```python
from build123d import *

# Parameters (mm, degrees)
SKETCH1_W           = 25
SKETCH1_H           = 40
BOSS_EXTRUDE1_DEPTH = 3
SKETCH2_W           = 3
SKETCH2_H           = 10
BOSS_EXTRUDE2_DEPTH = 3
SKETCH3_R           = 7.5
CUT_EXTRUDE1_DEPTH  = 4


with BuildPart() as part:
    # Sketch1 → Boss-Extrude1 (new body)
    with BuildSketch(Plane(origin=(0, 0, 0), x_dir=(1, 0, 0), z_dir=(0, 1, 0))):
        Rectangle(SKETCH1_W, SKETCH1_H)
    extrude(amount=BOSS_EXTRUDE1_DEPTH)

    # Sketch2 → Boss-Extrude2 (add)
    with BuildSketch(Plane(origin=(0, 3, 0), x_dir=(1, 0, 0), z_dir=(0, 1, 0))):
        with Locations((14, -15)):
            Rectangle(SKETCH2_W, SKETCH2_H)
        with Locations((14, 5)):
            Rectangle(SKETCH2_W, SKETCH2_H)
        with Locations((-14, -15)):
            Rectangle(SKETCH2_W, SKETCH2_H)
        with Locations((-14, 5)):
            Rectangle(SKETCH2_W, SKETCH2_H)
    extrude(amount=-BOSS_EXTRUDE2_DEPTH)

    # Sketch3 → Cut-Extrude1 (cut, through all)
    with BuildSketch(Plane(origin=(0, 3, 0), x_dir=(1, 0, 0), z_dir=(0, 1, 0))):
        with Locations((0, -7)):
            Circle(SKETCH3_R)
    extrude(amount=-CUT_EXTRUDE1_DEPTH, mode=Mode.SUBTRACT)


solid = part.part
```
For this review, take the finished solid that the model builds, in its own axes (mm). A direction names the side the tool comes from. Round coordinates to 2 decimals unless told otherwise and drop trailing zeros. Write each loop counter-clockwise with the first axis right and the second up, starting at its lowest first coordinate (ties: lowest second). Pieces come first, ordered by that corner, then holes. Notation, with made-up numbers: (71.5, 10) -> (92.5, 10) arc R17 ccw to (92.5, 43) -> close; hole circle Ø2 at (53, -29). An arc over 180 degrees is marked (long way). Use one line per item in the form item = value.
1) To check wall thickness, follow L1, parallel to Z at x = 0, y = 0.65; L2, parallel to X at y = 1.75, z = 7; L3, parallel to Z at x = -4, y = 2.1. State the ranges of each line that lie inside material, in increasing order. Write a range as from..to.
Found:
L1 = -20..-0.5, 14.5..20
L2 = -12.5..-7.5, 7.5..12.5
L3 = -20..0.66, 13.34..20
2) Take a section at C-C, the plane z = 7. Write out the cut boundary in (x, y), and give its area (3 significant figures).
Found:
outline = (-12.5, 0) -> (-7.5, 0) -> (-7.5, 3) -> (-12.5, 3) -> close; (7.5, 0) -> (12.5, 0) -> (12.5, 3) -> (7.5, 3) -> close
area = 30.0 mm2
3) Mouldability with a two-part tool opening along Z and no side actions: class faces 5 (the flat face through (-14, 2, 10)), 6 (the flat face through (0, 2, 20)), 7 (the flat face through (0, 3, -5)), 8 (the flat face through (14, 2, -10)) as +Z half, -Z half, draft (parallel to the pull), parting line (faces both ways), or undercut.
Found:
face_5 = undercut
face_6 = +Z half
face_7 = draft
face_8 = -Z half
4) Take a section at A-A, the plane x = 0. Write out the cut boundary in (y, z).
Found:
outline = (0, -20) -> (3, -20) -> (3, -0.5) -> (0, -0.5) -> close; (0, 14.5) -> (3, 14.5) -> (3, 20) -> (0, 20) -> close
5) Clearance check with flat-ended pins moving along their axes: pin 1 (0.9 mm diameter, centred on y = 1, z = 3.5, fed in from -X); pin 2 (1.5 mm diameter, centred on y = 1.5, z = -13, fed in from +X); pin 3 (0.9 mm diameter, centred on x = 14, y = 2, fed in from -Z). State where each tip first meets the part, or that it passes through.
Found:
pin_1 = -12.5
pin_2 = 12.5
pin_3 = -10
6) Tool access review of faces 1 (the flat face through (-14, 2, -10)), 2 (the flat face through (12.5, 1, 5)), 3 (the flat face through (-12.5, 1, 5)), 4 (the flat face through (12.5, 1, -15)): name each direction out of +Z, -Z, +X, -X, +Y, -Y from which nothing blocks a thin tool from reaching the whole face with its end or side.
Found:
face_1 = -Z, -X, +Y, -Y
face_2 = +X, +Y, -Y
face_3 = -X, +Y, -Y
face_4 = -Z, +X, +Y, -Y
7) Take a section at B-B, the plane y = 0.95. Write out the cut boundary in (x, z), and give its area (3 significant figures).
Found:
outline = (-15.5, -10) -> (-12.5, -10) -> (-12.5, -20) -> (12.5, -20) -> (12.5, -10) -> (15.5, -10) -> (15.5, 0) -> (12.5, 0) -> (12.5, 10) -> (15.5, 10) -> (15.5, 20) -> (-15.5, 20) -> (-15.5, 10) -> (-12.5, 10) -> (-12.5, 0) -> (-15.5, 0) -> close; hole circle Ø15 at (0, 7)
area = 943 mm2
